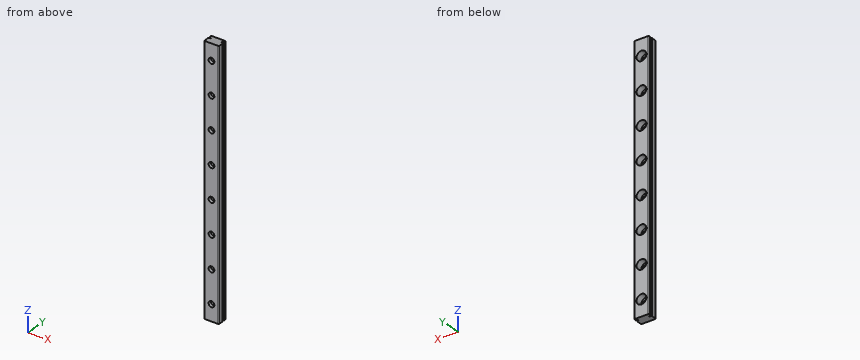
from build123d import *

# Parameters (mm, degrees)
BOSS_EXTRUDE1_DEPTH = 160
FILLET1_R           = 0.5
SKETCH2_R           = 3
CUT_EXTRUDE1_DEPTH  = 4
SKETCH3_R           = 1.75
CUT_EXTRUDE2_DEPTH  = 161.113241176
LPATTERN1_COUNT     = 8
LPATTERN1_PITCH     = 20


with BuildPart() as part:
    # Sketch1 → Boss-Extrude1 (new body)
    with BuildSketch(Plane.XY):
        Polygon((-4.5, 0), (4.5, 0), (4.5, 3.25), (3.1, 4), (4.5, 4.75), (4.5, 6), (-4.5, 6), (-4.5, 4.75), (-3.1, 4), (-4.5, 3.25), align=None)
    extrude(amount=BOSS_EXTRUDE1_DEPTH)

    # Fillet1
    fillet1_edges = [part.edges().sort_by_distance(p)[0] for p in [
        (-4.5, 6, 80),
        (4.5, 6, 80),
        (4.5, 0, 80),
        (-4.5, 0, 80),
    ]]
    fillet(fillet1_edges, radius=FILLET1_R)

    # Sketch2 → Cut-Extrude1 (cut)
    with BuildSketch(Plane(origin=(0, 6, 0), x_dir=(1, 0, 0), z_dir=(0, 1, 0))):
        with Locations(Location((0, -10, 0), (0, 0, 180))):
            Circle(SKETCH2_R)
    cut_extrude1 = extrude(amount=-CUT_EXTRUDE1_DEPTH, mode=Mode.SUBTRACT)

    # Sketch3 → Cut-Extrude2 (cut, through all)
    with BuildSketch(Plane(origin=(0, 2, 0), x_dir=(1, 0, 0), z_dir=(0, 1, 0))):
        with Locations(Location((0, -10, 0), (0, 0, 180))):
            Circle(SKETCH3_R)
    cut_extrude2 = extrude(amount=-CUT_EXTRUDE2_DEPTH, mode=Mode.SUBTRACT)

    # LPattern1: Cut-Extrude1, Cut-Extrude2 ×8
    with Locations(*[(0, 0, i * LPATTERN1_PITCH) for i in range(1, LPATTERN1_COUNT)]):
        add(cut_extrude1, mode=Mode.SUBTRACT)
        add(cut_extrude2, mode=Mode.SUBTRACT)


solid = part.part
Here's how the part is built. I have some questions about the finished solid (model axes, mm). Round coordinates to 2 decimals unless told otherwise and drop trailing zeros. Order: outer loops, then holes, each group sorted by start corner. A loop starts at its lowest first (then second) coordinate and runs counter-clockwise, first axis right, second up. Notation, with made-up numbers: M 31.5,68.5 L 56.5,68.5 A14 cw 56.5,81.5 Z; hole C -11,41 d9. An arc over 180 degrees is marked long. Return JSON: item names as keys, results as strings. Group by question number.
1. If we section it at B-B on x = 0: State how many separate pieces and enclosed holes the cut face has, then the cut area to 3 significant figures.
2. I'm going to push a flat-ended pin straight in: pin 1 Ø1.8 at (x, z) = (0, 109) entering from +Y. Where does the tip first touch, or does it pass through?
3. Please list where these lines run through material, in increasing order: probe 1 along X at (y, z) = (0.45, 130); probe 2 along X at (y, z) = (3.05, 90); probe 3 along Y at (x, z) = (4.25, 29).
4. If we section it at A-A on z = 110: List the corners of the cut face in (x, y) for me, then the cut area to 3 significant figures.
Reply:
{
 "1": {"separate pieces": "9", "enclosed holes": "0", "area": "712 mm^2"},
 "2": {"pin 1": "y = 2"},
 "3": {"probe 1": "-4.5 to -1.75, 1.75 to 4.5", "probe 2": "-4.5 to -3, 3 to 4.5", "probe 3": "0.07 to 3.38, 4.62 to 5.93"},
 "4": {"outline": "M -4.5,0.5 A0.5 ccw -4,0 L -1.75,0 L -1.75,2 L -3,2 L -3,6 L -4,6 A0.5 ccw -4.5,5.5 L -4.5,4.75 L -3.1,4 L -4.5,3.25 Z; M 1.75,0 L 4,0 A0.5 ccw 4.5,0.5 L 4.5,3.25 L 3.1,4 L 4.5,4.75 L 4.5,5.5 A0.5 ccw 4,6 L 3,6 L 3,2 L 1.75,2 Z", "area": "20.7 mm^2"}
}
